Could you check a few things on this model? Use its own coordinates, in mm. A direction names the side the tool comes from. Round coordinates to 2 decimals unless told otherwise and drop trailing zeros. Order: outer loops, then holes, each group sorted by start corner. A loop starts at its lowest first (then second) coordinate and runs counter-clockwise, first axis right, second up. Notation, with made-up numbers: (19, 8) - (36, 8) arc R12 cw to (36, 18) - close; hole circle Ø2 at (18.5, 71). An arc over 180 degrees is marked (long way). Return JSON: item names as keys, results as strings. Group by question number.
from build123d import *

# Parameters (mm, degrees)
BOSS_EXTRUDE1_DEPTH = 4
BOSS_EXTRUDE3_DEPTH = 2
BOSS_EXTRUDE4_DEPTH = 4
CUT_EXTRUDE1_DEPTH  = 4
BOSS_EXTRUDE6_START = -4
BOSS_EXTRUDE6_DEPTH = 4


with BuildPart() as part:
    # Sketch2 → Boss-Extrude1 (new body)
    with BuildSketch(Plane(origin=(0, 0, 0), x_dir=(1, 0, 0), z_dir=(0, 1, 0))):
        with BuildLine():
            Line((0.12816248, 0), (0.19140299, 0))
            Line((0.19140299, 0), (0.580035518, 0))
            Line((0.580035518, 0), (8, 0))
            Line((8, 0), (8.04118409, 0))
            ThreePointArc((8.04118409, 0), (13.15, 4.5), (18.25881591, 0))
            Line((18.25881591, 0), (18.3, 0))
            Line((18.3, 0), (26.3, 0))
            Line((26.3, 0), (27.90423081, 0))
            Line((27.90423081, 0), (42.8, 0))
            Line((42.8, 0), (52.528764428, 8.163402643))
            Line((52.528764428, 8.163402643), (42.8, 8.163402643))
            Line((42.8, 8.163402643), (42.8, 1.5))
            Line((42.8, 1.5), (26.3, 1.5))
            Line((26.3, 1.5), (26.3, 13.7))
            Line((26.3, 13.7), (-7.372368399, 13.7))
            Line((-7.372368399, 13.7), (-7.372368399, 5.162187927))
            Line((-7.372368399, 5.162187927), (0, 0))
            Line((0, 0), (0.12816248, 0))
        make_face()
        with BuildLine():
            ThreePointArc((18.25881591, 0), (13.15, 4.5), (8.04118409, 0))
            Line((8.04118409, 0), (8.088379706, 0))
            ThreePointArc((8.088379706, 0), (8.155534558, 0.306111042), (8.24118409, 0.607570661))
            ThreePointArc((8.24118409, 0.607570661), (10.108535624, 3.205958909), (13.15, 4.2))
            ThreePointArc((13.15, 4.2), (16.191464376, 3.205958909), (18.05881591, 0.607570661))
            ThreePointArc((18.05881591, 0.607570661), (18.144465442, 0.306111042), (18.211620294, 0))
            Line((18.211620294, 0), (18.25881591, 0))
        make_face()
        with BuildLine():
            ThreePointArc((13.15, 4.2), (10.108535624, 3.205958909), (8.24118409, 0.607570661))
            Line((8.24118409, 0.607570661), (8.24118409, 0))
            Line((8.24118409, 0), (13.15, 0))
            Line((13.15, 0), (13.15, 4.2))
        make_face()
        with BuildLine():
            ThreePointArc((18.05881591, 0.607570661), (16.191464376, 3.205958909), (13.15, 4.2))
            Line((13.15, 4.2), (13.15, 0))
            Line((13.15, 0), (18.05881591, 0))
            Line((18.05881591, 0), (18.05881591, 0.607570661))
        make_face()
        Polygon((13.15, 0), (8.24118409, 0), (8.24118409, -0.3), (18.05881591, -0.3), (18.05881591, 0), align=None)
        with BuildLine():
            ThreePointArc((8.24118409, 0.607570661), (8.155534558, 0.306111042), (8.088379706, 0))
            ThreePointArc((8.088379706, 0), (8.062570085, -0.14965204), (8.04118409, -0.3))
            Line((8.04118409, -0.3), (8.24118409, -0.3))
            Line((8.24118409, -0.3), (8.24118409, 0))
            Line((8.24118409, 0), (8.24118409, 0.607570661))
        make_face()
        with BuildLine():
            ThreePointArc((18.25881591, -0.3), (18.237429915, -0.14965204), (18.211620294, 0))
            ThreePointArc((18.211620294, 0), (18.144465442, 0.306111042), (18.05881591, 0.607570661))
            Line((18.05881591, 0.607570661), (18.05881591, 0))
            Line((18.05881591, 0), (18.05881591, -0.3))
            Line((18.05881591, -0.3), (18.25881591, -0.3))
        make_face()
        with BuildLine():
            Line((18.3, 0), (18.25881591, 0))
            Line((18.25881591, 0), (18.211620294, 0))
            ThreePointArc((18.211620294, 0), (18.237429915, -0.14965204), (18.25881591, -0.3))
            Line((18.25881591, -0.3), (42.8, -0.3))
            Line((42.8, -0.3), (42.992836283, -0.229813333))
            Line((42.992836283, -0.229813333), (43.639486744, 0.312790831))
            Line((43.639486744, 0.312790831), (52.721600711, 7.93358931))
            Line((52.721600711, 7.93358931), (52.528764428, 8.163402643))
            Line((52.528764428, 8.163402643), (42.8, 0))
            Line((42.8, 0), (27.90423081, 0))
            Line((27.90423081, 0), (26.3, 0))
            Line((26.3, 0), (18.3, 0))
        make_face()
        Polygon((-0.094589637, -0.3), (-7.54444133, 4.916442314), (-9.666674144, 1.88557975), (-1.261195156, -4), (0, -4), (42.8, -4), (45.371150439, -3.064177772), (55.099914866, 5.099224871), (52.721600711, 7.93358931), (43.639486744, 0.312790831), (42.992836283, -0.229813333), (42.8, -0.3), (18.25881591, -0.3), (18.05881591, -0.3), (8.24118409, -0.3), (8.04118409, -0.3), (0, -0.3), align=None)
        with BuildLine():
            Line((0.580035518, 0), (0.19140299, 0))
            Line((0.19140299, 0), (0.12816248, 0))
            Line((0.12816248, 0), (0, 0))
            Line((0, 0), (-7.372368399, 5.162187927))
            Line((-7.372368399, 5.162187927), (-7.54444133, 4.916442314))
            Line((-7.54444133, 4.916442314), (-0.094589637, -0.3))
            Line((-0.094589637, -0.3), (0, -0.3))
            Line((0, -0.3), (8.04118409, -0.3))
            ThreePointArc((8.04118409, -0.3), (8.062570085, -0.14965204), (8.088379706, 0))
            Line((8.088379706, 0), (8.04118409, 0))
            Line((8.04118409, 0), (8, 0))
            Line((8, 0), (0.580035518, 0))
        make_face()
    extrude(amount=BOSS_EXTRUDE1_DEPTH)

    # Sketch2_4 → Boss-Extrude3 (add)
    with BuildSketch(Plane(origin=(0, 0, 0), x_dir=(1, 0, 0), z_dir=(0, 1, 0))):
        Polygon((-0.094589637, -0.3), (-7.54444133, 4.916442314), (-9.666674144, 1.88557975), (-1.261195156, -4), (0, -4), (42.8, -4), (45.371150439, -3.064177772), (55.099914866, 5.099224871), (52.721600711, 7.93358931), (43.639486744, 0.312790831), (42.992836283, -0.229813333), (42.8, -0.3), (18.25881591, -0.3), (18.05881591, -0.3), (8.24118409, -0.3), (8.04118409, -0.3), (0, -0.3), align=None)
        with BuildLine():
            ThreePointArc((18.05881591, 0.607570661), (16.191464376, 3.205958909), (13.15, 4.2))
            Line((13.15, 4.2), (13.15, 0))
            Line((13.15, 0), (18.05881591, 0))
            Line((18.05881591, 0), (18.05881591, 0.607570661))
        make_face()
        with BuildLine():
            ThreePointArc((13.15, 4.2), (10.108535624, 3.205958909), (8.24118409, 0.607570661))
            Line((8.24118409, 0.607570661), (8.24118409, 0))
            Line((8.24118409, 0), (13.15, 0))
            Line((13.15, 0), (13.15, 4.2))
        make_face()
        Polygon((13.15, 0), (8.24118409, 0), (8.24118409, -0.3), (18.05881591, -0.3), (18.05881591, 0), align=None)
    extrude(amount=-BOSS_EXTRUDE3_DEPTH)

    # Sketch3 → Boss-Extrude4 (add)
    with BuildSketch(Plane(origin=(0, -2, 0), x_dir=(-1, 0, 0), z_dir=(0, -1, 0))):
        with BuildLine():
            Line((-18.25881591, 5.162187927), (-18.25881591, 0))
            ThreePointArc((-18.25881591, 0), (-13.15, 4.5), (-8.04118409, 0))
            Line((-8.04118409, 0), (-8, 0))
            Line((-8, 0), (-0.580035518, 0))
            Line((-0.580035518, 0), (-0.19140299, 0))
            Line((-0.19140299, 0), (-0.12816248, 0))
            Line((-0.12816248, 0), (0, 0))
            Line((0, 0), (7.372368399, 5.162187927))
            Line((7.372368399, 5.162187927), (-18.25881591, 5.162187927))
        make_face()
        Polygon((-52.528764428, 10.163402643), (-52.528764428, 8.163402643), (-44.028764428, 1.031055778), (-44.028764428, 8.163402643), (-44.028764428, 10.163402643), align=None)
        with BuildLine():
            Line((-44.028764428, 1.031055778), (-52.528764428, 8.163402643))
            Line((-52.528764428, 8.163402643), (-52.721600711, 7.93358931))
            Line((-52.721600711, 7.93358931), (-43.639486744, 0.312790831))
            Line((-43.639486744, 0.312790831), (-42.992836283, -0.229813333))
            Line((-42.992836283, -0.229813333), (-42.8, -0.3))
            Line((-42.8, -0.3), (-18.25881591, -0.3))
            ThreePointArc((-18.25881591, -0.3), (-18.237429915, -0.14965204), (-18.211620294, 0))
            Line((-18.211620294, 0), (-18.25881591, 0))
            Line((-18.25881591, 0), (-18.3, 0))
            Line((-18.3, 0), (-26.3, 0))
            Line((-26.3, 0), (-27.90423081, 0))
            Line((-27.90423081, 0), (-42.8, 0))
            Line((-42.8, 0), (-44.028764428, 1.031055778))
        make_face()
        Polygon((-43.639486744, 0.312790831), (-52.721600711, 7.93358931), (-55.099914866, 5.099224871), (-45.371150439, -3.064177772), (-42.8, -4), (0, -4), (1.261195156, -4), (9.666674144, 1.88557975), (7.54444133, 4.916442314), (0.094589637, -0.3), (0, -0.3), (-8.04118409, -0.3), (-8.24118409, -0.3), (-18.05881591, -0.3), (-18.25881591, -0.3), (-42.8, -0.3), (-42.992836283, -0.229813333), align=None)
        with BuildLine():
            Line((-13.15, 4.2), (-13.15, 0))
            Line((-13.15, 0), (-8.24118409, 0))
            Line((-8.24118409, 0), (-8.24118409, 0.607570661))
            ThreePointArc((-8.24118409, 0.607570661), (-10.108535624, 3.205958909), (-13.15, 4.2))
        make_face()
        with BuildLine():
            Line((-18.05881591, 0.607570661), (-18.05881591, 0))
            Line((-18.05881591, 0), (-13.15, 0))
            Line((-13.15, 0), (-13.15, 4.2))
            ThreePointArc((-13.15, 4.2), (-16.191464376, 3.205958909), (-18.05881591, 0.607570661))
        make_face()
        with BuildLine():
            Line((-8.24118409, 0), (-8.24118409, -0.3))
            Line((-8.24118409, -0.3), (-8.04118409, -0.3))
            ThreePointArc((-8.04118409, -0.3), (-8.062570085, -0.14965204), (-8.088379706, 0))
            ThreePointArc((-8.088379706, 0), (-8.155534558, 0.306111042), (-8.24118409, 0.607570661))
            Line((-8.24118409, 0.607570661), (-8.24118409, 0))
        make_face()
        Polygon((-18.05881591, 0), (-18.05881591, -0.3), (-8.24118409, -0.3), (-8.24118409, 0), (-13.15, 0), align=None)
        with BuildLine():
            Line((-8, 0), (-8.04118409, 0))
            Line((-8.04118409, 0), (-8.088379706, 0))
            ThreePointArc((-8.088379706, 0), (-8.062570085, -0.14965204), (-8.04118409, -0.3))
            Line((-8.04118409, -0.3), (0, -0.3))
            Line((0, -0.3), (0.094589637, -0.3))
            Line((0.094589637, -0.3), (7.54444133, 4.916442314))
            Line((7.54444133, 4.916442314), (7.372368399, 5.162187927))
            Line((7.372368399, 5.162187927), (0, 0))
            Line((0, 0), (-0.12816248, 0))
            Line((-0.12816248, 0), (-0.19140299, 0))
            Line((-0.19140299, 0), (-0.580035518, 0))
            Line((-0.580035518, 0), (-8, 0))
        make_face()
        with BuildLine():
            Line((-18.25881591, 0), (-18.211620294, 0))
            ThreePointArc((-18.211620294, 0), (-18.144465442, 0.306111042), (-18.05881591, 0.607570661))
            ThreePointArc((-18.05881591, 0.607570661), (-16.191464376, 3.205958909), (-13.15, 4.2))
            ThreePointArc((-13.15, 4.2), (-10.108535624, 3.205958909), (-8.24118409, 0.607570661))
            ThreePointArc((-8.24118409, 0.607570661), (-8.155534558, 0.306111042), (-8.088379706, 0))
            Line((-8.088379706, 0), (-8.04118409, 0))
            ThreePointArc((-8.04118409, 0), (-13.15, 4.5), (-18.25881591, 0))
        make_face()
        with BuildLine():
            ThreePointArc((-18.211620294, 0), (-18.237429915, -0.14965204), (-18.25881591, -0.3))
            Line((-18.25881591, -0.3), (-18.05881591, -0.3))
            Line((-18.05881591, -0.3), (-18.05881591, 0))
            Line((-18.05881591, 0), (-18.05881591, 0.607570661))
            ThreePointArc((-18.05881591, 0.607570661), (-18.144465442, 0.306111042), (-18.211620294, 0))
        make_face()
    extrude(amount=BOSS_EXTRUDE4_DEPTH)

    # Sketch4 → Cut-Extrude1 (cut)
    with BuildSketch(Plane(origin=(0, -6, 0), x_dir=(-1, 0, 0), z_dir=(0, -1, 0))):
        Polygon((-18.25881591, 0), (-12.25881591, 0), (-12.25881591, 5.162187927), (-18.25881591, 5.190707464), align=None)
    extrude(amount=-CUT_EXTRUDE1_DEPTH, mode=Mode.SUBTRACT)

    # Sketch5 → Boss-Extrude6 (add)
    with BuildSketch(Plane(origin=(0, -6, 0), x_dir=(-1, 0, 0), z_dir=(0, -1, 0)).offset(BOSS_EXTRUDE6_START)):
        with BuildLine():
            Line((-18.05881591, 0), (-18.05881591, 0.607570661))
            ThreePointArc((-18.05881591, 0.607570661), (-15.819022848, 3.454408818), (-12.25881591, 4.122306272))
            Line((-12.25881591, 4.122306272), (-12.25881591, 0))
            Line((-12.25881591, 0), (-18.05881591, 0))
        make_face()
    extrude(amount=BOSS_EXTRUDE6_DEPTH)


solid = part.part
1) If I drill on line 1 along X through (y, z) = (-4.5, -9.75); line 2 along Y through (x, z) = (1.5, -2.75); line 3 along Y through (x, z) = (21.5, -11), over which ranges is the centre line in solid material (lowest first)? Write a range as from..to.
2) We'd pull the mould along X, two halves only. Please class faces 1 (the flat face through (-5.4, -0.9, 1.1)), 2 (the flat face through (44.104, -0.93, 3.526)), 3 (the flat face through (30, -4, 0)), 4 (the flat face through (21, -1, 4)): +X half, -X half, draft (parallel to the pull), parting line (faces both ways), or undercut.
3) I want a section at A-A, the plane z = -3.25. List the corners of the cut face in (x, y) for me, plus the area to 3 significant figures.
4) I want a section at D-D, the plane y = -3.25. List the corners of the cut face in (x, z) for me.
5) I want a section at C-C, the plane y = 1.75. List the corners of the cut face in (x, z) for me, plus the area to 3 significant figures.
6) I want a section at B-B, the plane x = 2.5. List the corners of the cut face in (y, z) for me.
7) Will these pins go through, and if not, where does the flat tip stop? pin 1 (2 mm diameter, centred on y = 2.5, z = -4, fed in from -X); pin 2 (4.5 mm diameter, centred on y = 1, z = -11, fed in from -X); pin 3 (4.5 mm diameter, centred on x = 49, y = -4.5, fed in from -Z).
8) For faces 5 (the flat face through (2, -2, -3)), 6 (the flat face through (52.529, -4, -9)), 7 (the flat face through (2, -4, -5.162)), 8 (the flat face through (42.8, 2, -5)), which set-ups out of +Z, -Z, +X, -X, +Y, -Y let a thin tool reach every point of the face, with its end or its side?
Outcome:
{
 "1": {"line 1": "44.03..52.53", "line 2": "-6..-2, 0..4", "line 3": "0..4"},
 "2": {"face 1": "-X half", "face 2": "+X half", "face 3": "undercut", "face 4": "draft"},
 "3": {"outline": "(-8.71, -6) - (16.13, -6) - (16.13, 0) - (26.3, 0) - (26.3, 4) - (-8.71, 4) - close; (42.8, 0) - (47.14, 0) - (47.14, -2) - (44.03, -2) - (44.03, -6) - (52.9, -6) - (52.9, 4) - (42.8, 4) - close; hole (-5.16, -2) - (10.17, -2) - (10.17, 0) - (-5.16, 0) - close", "area": "346 mm^2"},
 "4": {"outline": "(-9.67, -1.89) - (-7.37, -5.16) - (12.26, -5.16) - (12.26, -4.12) arc R5.15 ccw to (18.06, -0.61) - (18.06, 0) - (42.8, 0) - (44.03, -1.03) - (44.03, -10.16) - (52.53, -10.16) - (52.53, -8.16) - (55.1, -5.1) - (45.37, 3.06) - (42.8, 4) - (-1.26, 4) - close"},
 "5": {"outline": "(-9.67, -1.89) - (-7.37, -5.16) - (-7.37, -13.7) - (26.3, -13.7) - (26.3, -1.5) - (42.8, -1.5) - (42.8, -8.16) - (52.53, -8.16) - (55.1, -5.1) - (45.37, 3.06) - (42.8, 4) - (-1.26, 4) - close", "area": "775 mm^2"},
 "6": {"outline": "(-6, -5.16) - (-2, -5.16) - (-2, 0.3) - (0, 0.3) - (0, -13.7) - (4, -13.7) - (4, 4) - (-6, 4) - close"},
 "7": {"pin 1": "x = -8.89", "pin 2": "x = -7.37", "pin 3": "z = -10.16"},
 "8": {"face 5": "-Z", "face 6": "-Z, +X, +Y, -Y", "face 7": "-Z, -X, -Y", "face 8": "-Z, +Y, -Y"}
}
